For this review, take the finished solid that the model builds, in its own axes (mm). Face numbers are marked on the shaded views. Give positions to 0.01 mm unless a question says otherwise; leave off trailing zeros. Use CSV: the item, a comma, the result in double quotes. Start each with the question number.
1. Take a section at A-A on z = 1.35. State how many separate pieces and enclosed holes the cut face has, plus the area to 3 significant figures.
2. For pin 1 (3.5 mm diameter, centred on x = 37.91, y = 21.88, fed in from +Z), flat-tipped, find the tip position at first contact; note if it passes through.
3. Wall thickness on line 1 (Y direction, x = -6, z = 2.25); line 2 (X direction, y = -43, z = 1.9); line 3 (X direction, y = 16.5, z = 0.5): over which ranges is each line inside the solid? List them lowest first.
4. Mouldability with a two-part tool opening along Z and no side actions: class the marked faces 1 and 2 as pulls with the +Z half, pulls with the -Z half, needs draft (parallel to the pull), parting line crosses it, or undercut.
```python
from build123d import *

# Parameters (mm, degrees)
F1_DEPTH = 3
F2_R     = 4.6
F3_DEPTH = 25
F4_R     = 1.6946230943
F4_R_2   = 1.5
F5_DEPTH = 30


with BuildPart() as f1:
    # F0 (on Top) → F1 (new body)
    with BuildSketch(Plane.XY):
        with BuildLine():
            Line((-6.75, 29.5), (-6.75, 18.8265105636))
            ThreePointArc((-6.75, 18.8265105636), (-10.705427356, 16.893603083), (-14.1421356237, 14.1421356237))
            ThreePointArc((-14.1421356237, 14.1421356237), (-16.893603083, 10.705427356), (-18.8265105636, 6.75))
            Line((-18.8265105636, 6.75), (-42.5142997889, 20.3221463664))
            ThreePointArc((-42.5142997889, 20.3221463664), (-47.5071396994, 20.3097918389), (-50, 15.983794783))
            Line((-50, 15.983794783), (-50, -25.3888497949))
            Line((-50, -25.3888497949), (-34.5, -25.3888497949))
            Line((-34.5, -25.3888497949), (-34.5, -11.75))
            ThreePointArc((-34.5, -11.75), (-33.0355339059, -8.2144660941), (-29.5, -6.75))
            Line((-29.5, -6.75), (-18.8265105636, -6.75))
            ThreePointArc((-18.8265105636, -6.75), (-16.893603083, -10.705427356), (-14.1421356237, -14.1421356237))
            ThreePointArc((-14.1421356237, -14.1421356237), (-10.705427356, -16.893603083), (-6.75, -18.8265105636))
            Line((-6.75, -18.8265105636), (-20.3221463664, -42.5142997889))
            ThreePointArc((-20.3221463664, -42.5142997889), (-20.3097918389, -47.5071396994), (-15.983794783, -50))
            Line((-15.983794783, -50), (25.3888497949, -50))
            Line((25.3888497949, -50), (25.3888497949, -34.5))
            Line((25.3888497949, -34.5), (11.75, -34.5))
            ThreePointArc((11.75, -34.5), (8.2144660941, -33.0355339059), (6.75, -29.5))
            Line((6.75, -29.5), (6.75, -18.8265105636))
            ThreePointArc((6.75, -18.8265105636), (10.705427356, -16.893603083), (14.1421356237, -14.1421356237))
            ThreePointArc((14.1421356237, -14.1421356237), (16.893603083, -10.705427356), (18.8265105636, -6.75))
            Line((18.8265105636, -6.75), (42.5142997889, -20.3221463664))
            ThreePointArc((42.5142997889, -20.3221463664), (47.5071396994, -20.3097918389), (50, -15.983794783))
            Line((50, -15.983794783), (50, 25.3888497949))
            Line((50, 25.3888497949), (34.5, 25.3888497949))
            Line((34.5, 25.3888497949), (34.5, 11.75))
            ThreePointArc((34.5, 11.75), (33.0355339059, 8.2144660941), (29.5, 6.75))
            Line((29.5, 6.75), (18.8265105636, 6.75))
            ThreePointArc((18.8265105636, 6.75), (16.893603083, 10.705427356), (14.1421356237, 14.1421356237))
            ThreePointArc((14.1421356237, 14.1421356237), (10.705427356, 16.893603083), (6.75, 18.8265105636))
            Line((6.75, 18.8265105636), (20.3221463664, 42.5142997889))
            ThreePointArc((20.3221463664, 42.5142997889), (20.3097918389, 47.5071396994), (15.983794783, 50))
            Line((15.983794783, 50), (-25.3888497949, 50))
            Line((-25.3888497949, 50), (-25.3888497949, 34.5))
            Line((-25.3888497949, 34.5), (-11.75, 34.5))
            ThreePointArc((-11.75, 34.5), (-8.2144660941, 33.0355339059), (-6.75, 29.5))
        make_face()
        with BuildLine():
            ThreePointArc((-7.7781745931, 7.7781745931), (0, 11), (7.7781745931, 7.7781745931))
            ThreePointArc((7.7781745931, 7.7781745931), (11, 0), (7.7781745931, -7.7781745931))
            ThreePointArc((7.7781745931, -7.7781745931), (0, -11), (-7.7781745931, -7.7781745931))
            ThreePointArc((-7.7781745931, -7.7781745931), (-11, 0), (-7.7781745931, 7.7781745931))
        make_face(mode=Mode.SUBTRACT)
    extrude(amount=F1_DEPTH)

    # F2 (on Top) → F3 (cut)
    with BuildSketch(Plane.XY):
        with Locations((-14.8245864651, 42.2937068045)):
            Circle(F2_R)
        with Locations((-2.9845864651, 42.2937068045)):
            Circle(F2_R)
        with Locations((8.8554135349, 42.2937068045)):
            Circle(F2_R)
        with Locations((-42.2937068045, -2.9845864651)):
            Circle(F2_R)
        with Locations((-42.2937068045, 8.8554135349)):
            Circle(F2_R)
        with Locations((-42.2937068045, -14.8245864651)):
            Circle(F2_R)
        with Locations((2.9845864651, -42.2937068045)):
            Circle(F2_R)
        with Locations((-8.8554135349, -42.2937068045)):
            Circle(F2_R)
        with Locations((14.8245864651, -42.2937068045)):
            Circle(F2_R)
        with Locations((42.2937068045, 2.9845864651)):
            Circle(F2_R)
        with Locations((42.2937068045, -8.8554135349)):
            Circle(F2_R)
        with Locations((42.2937068045, 14.8245864651)):
            Circle(F2_R)
    extrude(amount=F3_DEPTH, mode=Mode.SUBTRACT)

    # F4 (on Top) → F5 (cut)
    with BuildSketch(Plane.XY):
        with Locations((16.7920645326, 45.6192344427)):
            Circle(F4_R)
        with Locations((-21.8333657831, 47.1258349717)):
            Circle(F4_R_2)
        with Locations((-21.8763593584, 37.9076637328)):
            Circle(F4_R_2)
        with Locations((8.9827191732, 32.5078293681)):
            Circle(F4_R_2)
        with Locations((0, 17.4654945731)):
            Circle(F4_R_2)
        with Locations((-2.5026722487, 32.5078293681)):
            Circle(F4_R_2)
        with Locations((-32.5078293681, -2.5026722487)):
            Circle(F4_R_2)
        with Locations((-37.9076637328, -21.8763593584)):
            Circle(F4_R_2)
        with Locations((-45.6192344427, 16.7920645326)):
            Circle(F4_R)
        with Locations((-32.5078293681, 8.9827191732)):
            Circle(F4_R_2)
        with Locations((-47.1258349717, -21.8333657831)):
            Circle(F4_R_2)
        with Locations((-17.4654945731, 0)):
            Circle(F4_R_2)
        with Locations((2.5026722487, -32.5078293681)):
            Circle(F4_R_2)
        with Locations((21.8763593584, -37.9076637328)):
            Circle(F4_R_2)
        with Locations((-16.7920645326, -45.6192344427)):
            Circle(F4_R)
        with Locations((-8.9827191732, -32.5078293681)):
            Circle(F4_R_2)
        with Locations((21.8333657831, -47.1258349717)):
            Circle(F4_R_2)
        with Locations((0, -17.4654945731)):
            Circle(F4_R_2)
        with Locations((32.5078293681, 2.5026722487)):
            Circle(F4_R_2)
        with Locations((37.9076637328, 21.8763593584)):
            Circle(F4_R_2)
        with Locations((45.6192344427, -16.7920645326)):
            Circle(F4_R)
        with Locations((32.5078293681, -8.9827191732)):
            Circle(F4_R_2)
        with Locations((47.1258349717, 21.8333657831)):
            Circle(F4_R_2)
        with Locations((17.4654945731, 0)):
            Circle(F4_R_2)
    extrude(amount=F5_DEPTH, mode=Mode.SUBTRACT)


solid = f1.part
```
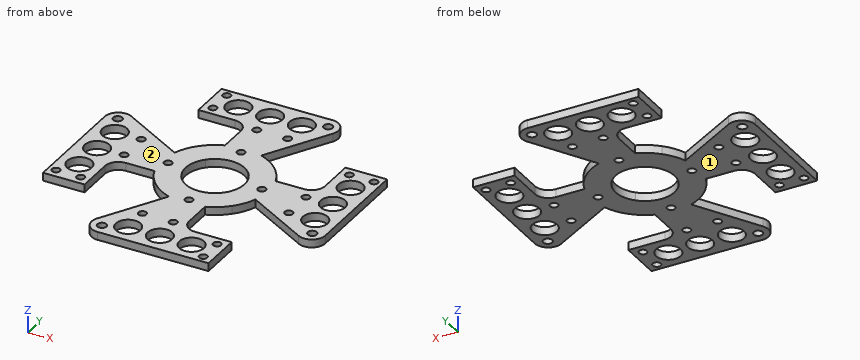
Check result:
1,separate pieces,"1"
1,enclosed holes,"37"
1,area,"3,760 mm²"
2,pin 1,"stops at z = 3"
3,line 1,"y = -50 to -45.9, -38.69 to -9.22, 9.22 to 38.82, 45.77 to 50"
3,line 2,"x = -20.57 to -13.4, -4.31 to -1.56, 7.53 to 10.28, 19.37 to 25.39"
3,line 3,"x = -49.97 to -47.29, -43.95 to -35.84, -11.3 to -1.15, 1.15 to 11.3, 34.5 to 38.01, 46.58 to 50"
4,face 1,"pulls with the -Z half"
4,face 2,"pulls with the +Z half"
